from build123d import *

# Parameters (mm, degrees)
SKETCH1_R           = 1.5875
BOSS_EXTRUDE1_DEPTH = 6.35


with BuildPart() as part:
    # Sketch1 → Boss-Extrude1 (new body)
    with BuildSketch(Plane.XY):
        with BuildLine():
            Line((10.795, 0), (10.795, 10.795))
            Line((10.795, 10.795), (23.495, 10.795))
            Line((23.495, 10.795), (23.495, 14.605))
            Line((23.495, 14.605), (-10.795, 14.605))
            Line((-10.795, 14.605), (-10.795, 0))
            ThreePointArc((-10.795, 0), (0, -10.795), (10.795, 0))
        make_face()
        Circle(SKETCH1_R, mode=Mode.SUBTRACT)
        with Locations((-4.95, 4.95)):
            Circle(SKETCH1_R, mode=Mode.SUBTRACT)
        with Locations((-4.95, -4.95)):
            Circle(SKETCH1_R, mode=Mode.SUBTRACT)
        with Locations((4.95, -4.95)):
            Circle(SKETCH1_R, mode=Mode.SUBTRACT)
        with Locations((4.95, 4.95)):
            Circle(SKETCH1_R, mode=Mode.SUBTRACT)
    extrude(amount=BOSS_EXTRUDE1_DEPTH)


solid = part.part
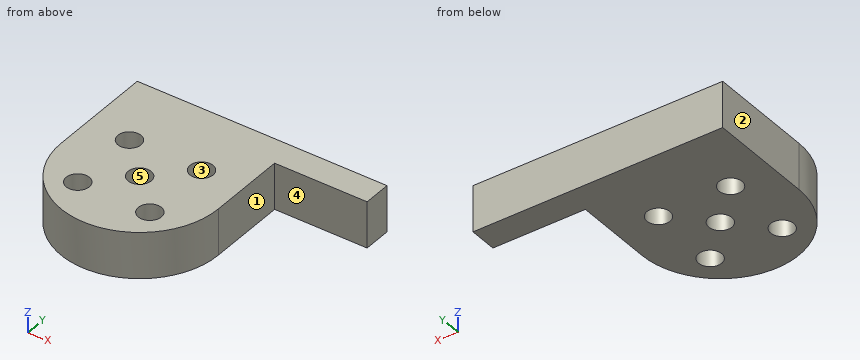
Input: part model. Units: mm. Frame: model coordinates. Face numbers are marked on the shaded views. A direction names the side the tool comes from. Coordinates: 2 decimals unless noted, no trailing zeros. Order: outer loops, then holes, each group sorted by start corner. A loop starts at its lowest first (then second) coordinate and runs counter-clockwise, first axis right, second up.
1. Ray query, line 1 along Y through (x, z) = (0, 2.5) (1 decimal); line 2 along X through (y, z) = (-6, 5); line 3 along Y through (x, z) = (-4.95, 1.75) (1 decimal). Return the intervals inside material, ascending.
Checked values:
line 1: y = -10.8 to -1.6, 1.6 to 14.6
line 2: x = -8.97 to -6.14, -3.76 to 3.76, 6.14 to 8.97
line 3: y = -9.6 to -6.5, -3.4 to 3.4, 6.5 to 14.6
2. Cut plane D-D, the plane x = -6. Return loops of the section in (y, z) (3 decimals).
Checked values:
outline: (-8.974, 0) - (-6.141, 0) - (-6.141, 6.35) - (-8.974, 6.35) - close; (-3.759, 0) - (3.759, 0) - (3.759, 6.35) - (-3.759, 6.35) - close; (6.141, 0) - (14.605, 0) - (14.605, 6.35) - (6.141, 6.35) - close
3. Cut plane B-B, the plane y = 4.95. Count the separate pieces of the cut face and the enclosed holes in it, plus the area to 3 significant figures.
Checked values:
separate pieces: 3
enclosed holes: 0
area: 96.8 mm2
4. Draft query along X for the marked faces 1, 2 and 3. Return one class per face: +X half, -X half, draft (parallel to the pull), parting line (faces both ways), or undercut.
Checked values:
face 1: +X half
face 2: -X half
face 3: undercut
5. Access query for the marked faces 4 and 5. Directions: +Z, -Z, +X, -X, +Y, -Y. A direction counts if a zero-diameter tool reaches every point of the face in a straight line with its end or side. Return the directions, or none.
Checked values:
face 4: +Z, -Z, +X, -Y
face 5: +Z, -Z
6. Contact query for flat-ended pins moving along their axis: P1, Ø1.9, axis at x = 0, y = 0, coming from the -Z side; P2, Ø3, axis at x = 16.5, z = 3.5, coming from the -Y side (3 decimals). Output: stop coordinate, or through.
Checked values:
P1: passes through
P2: stops at y = 10.795
